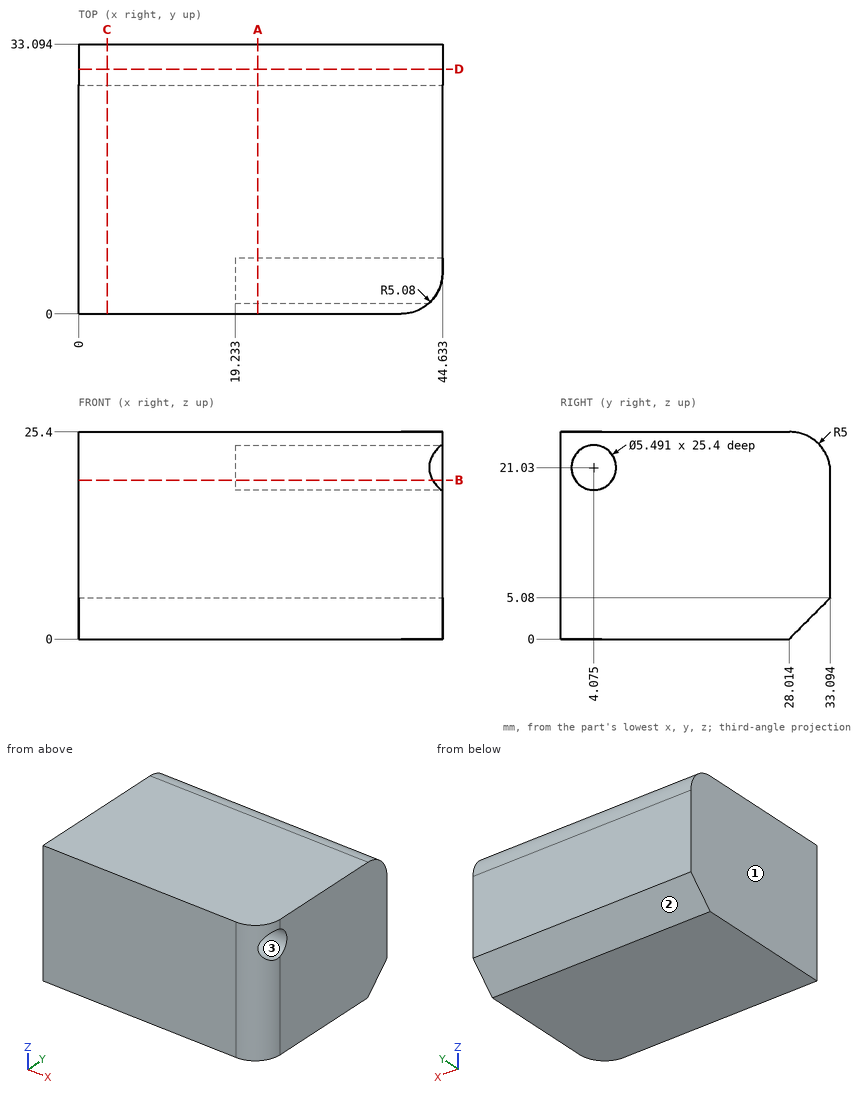
Check sheet for the drawn part. Datum: minimum x, y, z corner. Units: mm. Round coordinates to 2 decimals unless told otherwise and drop trailing zeros. Order: outer loops, then holes, each group sorted by start corner. A loop starts at its lowest first (then second) coordinate and runs counter-clockwise, first axis right, second up. Notation, with made-up numbers: (25.25, 1) -> (62.25, 1) arc R35 cw to (62.25, 37) -> close; hole circle Ø6 at (-18.5, 35). An arc over 180 degrees is marked (long way). Put each result on its own line as item: value. Start each with the question number.
(1) Section check A-A (x = 22). Enter the section's corners in (y, z) (1 decimal), then the cut area to 3 significant figures.
(2) Section check C-C (x = 3.5). Enter the section's corners in (y, z) (1 decimal), then the cut area to 3 significant figures.
(3) Draft check along Z on the marked faces 1, 2 and 3. Enter one of: +Z half, -Z half, draft (parallel to the pull), parting line (faces both ways), or undercut.
(4) Section check B-B (z = 19.5). Enter the section's corners in (x, y) (1 decimal).
(5) Depth check by flat-ended pin: pin 1 Ø1.6 at (y, z) = (5.5, 21.5) entering from +X. Enter the tip coordinate at first touch or a pass-through.
(6) Section check D-D (y = 30). Enter the section's corners in (x, z) (1 decimal).
(7) Material ranges on line 1 along Y through (x, z) = (33.5, 20.25) (1 decimal); line 2 along Y through (x, z) = (26, 2.5) (1 decimal); line 3 along Z through (x, y) = (31.5, 5) (1 decimal), recorded low to high.
Completed:
1. outline: (0, 0) -> (28, 0) -> (33.1, 5.1) -> (33.1, 20.4) arc R5 ccw to (28.1, 25.4) -> (0, 25.4) -> close; hole circle Ø5.5 at (4.1, 21)
1. area: 799 mm2
2. outline: (0, 0) -> (28, 0) -> (33.1, 5.1) -> (33.1, 20.4) arc R5 ccw to (28.1, 25.4) -> (0, 25.4) -> close
2. area: 822 mm2
3. face 1: draft
3. face 2: -Z half
3. face 3: undercut
4. outline: (0, 0) -> (39.6, 0) arc R5.1 ccw to (43.4, 1.8) -> (19.2, 1.8) -> (19.2, 6.4) -> (44.6, 6.4) -> (44.6, 33.1) -> (0, 33.1) -> close
5. pin 1: stops at x = 19.23
6. outline: (0, 2) -> (44.6, 2) -> (44.6, 25) -> (0, 25) -> close
7. line 1: y = 0 to 1.4, 6.7 to 33.1
7. line 2: y = 0 to 30.5
7. line 3: z = 0 to 18.4, 23.6 to 25.4
